Answer from the drawing. Dimensions are ordinates in mm from the lowest x, y and z of the part. A direction names the side the tool comes from. Give positions to 0.01 mm unless a question says otherwise; leave off trailing zeros. Write each loop counter-clockwise with the first axis right and the second up, starting at its lowest first coordinate (ties: lowest second). Pieces come first, ordered by that corner, then holes. Notation, with made-up numbers: (45.5, 37.25) -> (49.5, 37.25) arc R24 cw to (49.5, 58.25) -> close; hole circle Ø2 at (26.5, 12). An arc over 180 degrees is marked (long way). Put each result on its own line as item: value. Start each with the question number.
1) For the marked faces 1 and 2, determine the directions among +Z, -Z, +X, -X, +Y, -Y from which every point of the face is accessible in a straight line to the end or side of a thin tool.
2) A cutting plane is placed at B-B (y = 12.5). Write down the section's boundary in (x, z) (1 decimal).
3) For a pull along Z with two mould halves and no side action, classify the marked faces 3, 4 and 5 as released by +Z, released by -Z, zero draft, split by the parting line, or undercut.
4) A cutting plane is placed at D-D (x = 56.5). Write down the section's boundary in (y, z) (1 decimal).
5) A cutting plane is placed at C-C (x = 14.5). Write down the section's boundary in (y, z).
6) Find the intervals of material crossed by line 1 along Z through (x, y) = (46, 68.5); line 2 along X through (y, z) = (7.5, 29.5) (1 decimal); line 3 along Y through (x, z) = (3.5, 5.5) (1 decimal), in increasing order. Write a range as from..to.
7) Flat-ended cylindrical pins translate along their axes: pin 1 Ø8 at (y, z) = (66, 26) entering from +X; pin 2 Ø10 at (x, z) = (20, 35) entering from -Y (1 decimal). Find the tip coordinate at first contact, or state that the pin passes through.
8) A cutting plane is placed at A-A (z = 30.5). Write down the section's boundary in (x, y).
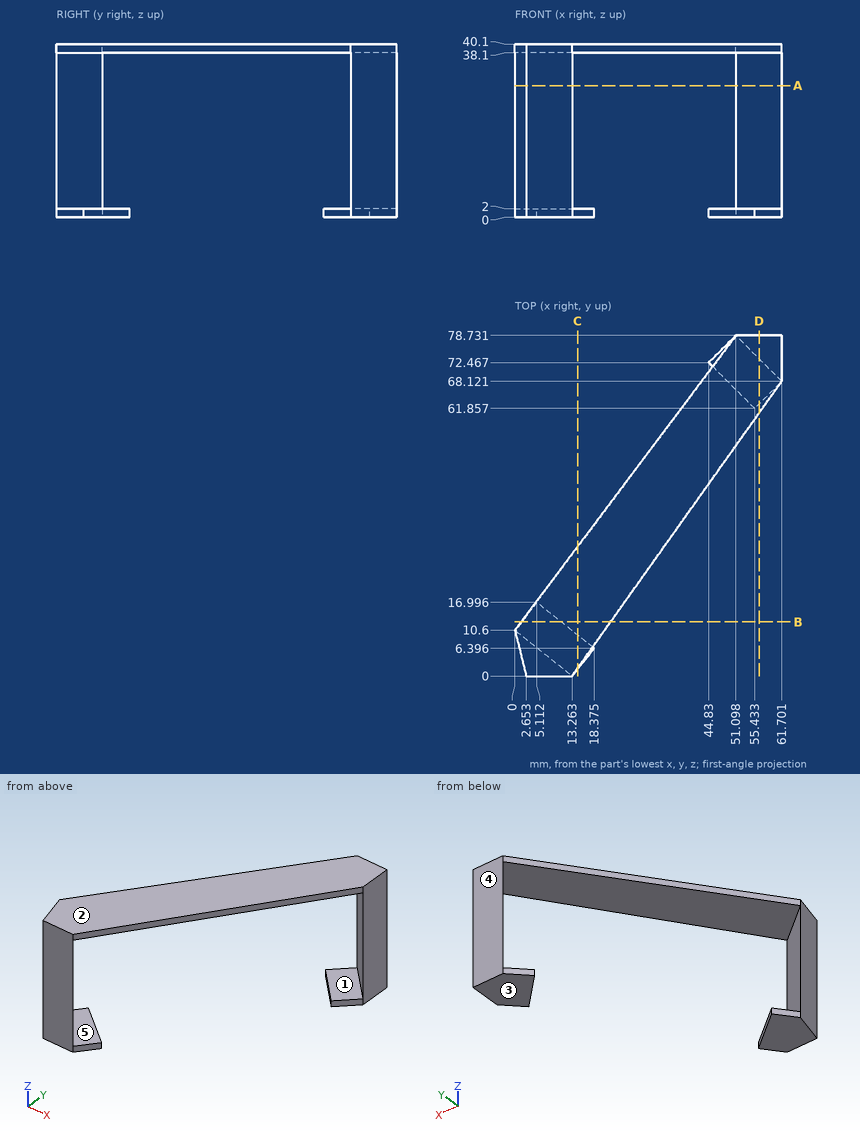
Reply:
1. face 1: -X, -Y
1. face 2: +Z, +X, -X, +Y, -Y
2. outline: (1.4, 38.1) -> (22.2, 38.1) -> (22.2, 40.1) -> (1.4, 40.1) -> close; (1.5, 0) -> (10.7, 0) -> (10.7, 2) -> (1.5, 2) -> close
3. face 3: released by -Z
3. face 4: zero draft
3. face 5: undercut
4. outline: (60.8, 38.1) -> (73.3, 38.1) -> (73.3, 2) -> (62.9, 2) -> (62.9, 0) -> (78.7, 0) -> (78.7, 40.1) -> (60.8, 40.1) -> close
5. outline: (1.55, 0) -> (9.49, 0) -> (9.49, 2) -> (1.55, 2) -> close; (1.74, 38.1) -> (29.93, 38.1) -> (29.93, 40.1) -> (1.74, 40.1) -> close
6. line 1: z = 38.1..40.1
6. line 2: x = 0.8..3.9
6. line 3: y = 0..7.8
7. pin 1: stops at x = 61.7
7. pin 2: stops at y = 4
8. outline: (0, 10.6) -> (2.65, 0) -> (13.26, 0) -> close; (51.1, 78.73) -> (61.7, 68.12) -> (61.7, 78.73) -> close
